Design review of the part built by this model. Coordinates are the model's own, in mm. A direction names the side the tool comes from. Coordinates: 2 decimals unless noted, no trailing zeros. Loops run counter-clockwise (first coordinate to the right, second up) from the corner with the lowest first, then second, coordinate; pieces in that order, holes last. Notation, with made-up numbers: (-10, -31.5) - (27, -31.5) arc R4 ccw to (27, -26.5) - close; hole circle Ø11 at (65, 54). An arc over 180 degrees is marked (long way). One line per question, with ' | ' between items.
from build123d import *

# Parameters (mm, degrees)
F1_DEPTH = 112.526558


with BuildPart() as f1:
    # F0 (on Front) → F1 (new body)
    with BuildSketch(Plane.XZ):
        with BuildLine():
            Line((38.495421, -30.370116), (45.421928, 37.163377))
            ThreePointArc((45.421928, 37.163377), (0.635948, 61.819784), (-44.223107, 37.296578))
            Line((-44.223107, 37.296578), (-44.223107, -0.875685))
            ThreePointArc((-44.223107, -0.875685), (-10.598014, 4.062906), (7.804978, -24.509221))
            ThreePointArc((7.804978, -24.509221), (7.564505, -28.386732), (6.846773, -32.204817))
            Line((6.846773, -32.204817), (38.495421, -30.370116))
        make_face()
        with BuildLine():
            ThreePointArc((7.804978, -24.509221), (-10.598014, 4.062906), (-44.223107, -0.875685))
            Line((-44.223107, -0.875685), (-44.223107, -35.165384))
            Line((-44.223107, -35.165384), (6.846773, -32.204817))
            ThreePointArc((6.846773, -32.204817), (7.564505, -28.386732), (7.804978, -24.509221))
        make_face()
        with BuildLine():
            Line((-44.223107, -35.165384), (-44.223107, -0.875685))
            ThreePointArc((-44.223107, -0.875685), (-39.986448, -51.258757), (6.846773, -32.204817))
            Line((6.846773, -32.204817), (-44.223107, -35.165384))
        make_face()
    extrude(amount=F1_DEPTH)


solid = f1.part
Q1. Draft analysis for pull direction X (two halves, no side actions). For faces 3 (the cylindrical face through (1.383, -55.476, 61.813)), 4 (the flat face through (-5, 0, 4)), 5 (the flat face through (22.45, -55.48, -31.3)), state which applies: +X half, -X half, draft (parallel to the pull), parting line (faces both ways), or undercut.
Returned:
face 3: parting line | face 4: draft | face 5: +X half
Q2. Take a section at A-A (y = -36.5). Give the boundary of the cut face in (x, z), plus the area to 3 significant figures.
Returned:
outline: (-44.22, -0.88) arc R31.38 ccw (long way) to (6.85, -32.2) - (38.5, -30.37) - (45.42, 37.16) arc R53.15 ccw to (-44.22, 37.3) - close | area: 8,830 mm²
Q3. To check wall thickness, follow line 1 along Z through (x, y) = (-36, -48); line 2 along X through (y, z) = (-22, 6); line 3 along Z through (x, y) = (-51, -76). State the ranges of each line that lie inside material, in increasing order.
Returned:
line 1: z = -53.33 to 47.25 | line 2: x = -44.22 to 42.23 | line 3: z = -39.77 to -9.25
Q4. For pin 1 (10 mm diameter, centred on y = -45, z = -12.5, fed in from +X); pin 2 (5 mm diameter, centred on y = -59.5, z = -26, fed in from +X); pin 3 (12 mm diameter, centred on x = 19, y = -60, fed in from +Z), all flat-tipped, find the tip position at first contact; note any pin that passes through.
Returned:
pin 1: stops at x = 40.84 | pin 2: stops at x = 39.2 | pin 3: stops at z = 60.34
Q5. Take a section at C-C (x = 29). Give the boundary of the cut face in (y, z), plus the area to 3 significant figures.
Returned:
outline: (-112.53, -30.92) - (0, -30.92) - (0, 53.57) - (-112.53, 53.57) - close | area: 9,510 mm²
Q6. Tool access review of faces 1 (the flat face through (-5, -112.527, 4)), 2 (the flat face through (-44.223, -55, 18)): name each direction out of +Z, -Z, +X, -X, +Y, -Y from which nothing blocks a thin tool from reaching the whole face with its end or side.
Returned:
face 1: +Z, -Z, +X, -X, -Y | face 2: +Z, -X, +Y, -Y
Q7. Take a section at B-B (z = -21). Give the boundary of the cut face in (x, y), plus the area to 3 significant figures.
Returned:
outline: (-54.76, -112.53) - (39.46, -112.53) - (39.46, 0) - (-54.76, 0) - close | area: 10,600 mm²
